Answer from the drawing. Dimensions are ordinates in mm from the lowest x, y and z of the part. A direction names the side the tool comes from. Coordinates: 2 decimals unless noted, no trailing zeros. Write each loop counter-clockwise with the first axis right and the second up, starting at its lowest first coordinate (ties: lowest second). Pieces come first, ordered by that corner, then holes. Notation, with made-up numbers: (36.5, 45.25) - (42.5, 45.25) arc R21 cw to (42.5, 56.25) - close; hole circle Ø6 at (-16, 29.5). An arc over 180 degrees is marked (long way). Use one line per item in the form item = value. Start each with the question number.
Item 1: A cutting plane is placed at D-D (z = 4). Write down the section's boundary in (x, y), then the cut area to 3 significant figures.
Item 2: Given pin 1 (4.5 mm diameter, centred on x = 6.5, y = 21.5, fed in from -Z); pin 2 (3.5 mm diameter, centred on x = 30.13, z = 32, fed in from -Y); pin 3 (5 mm diameter, centred on x = 28.5, z = 15.5, fed in from +Y); pin 4 (5 mm diameter, centred on y = 24, z = 29, fed in from +X), each flat-ended and moving along its own axis, determine where each tip first touches the part or whether it passes through.
Item 3: For the marked faces 4, 5 and 6, determine the directions among +Z, -Z, +X, -X, +Y, -Y from which every point of the face is accessible in a straight line to the end or side of a thin tool.
Item 4: A cutting plane is placed at B-B (x = 14). Write down the section's boundary in (y, z), then the cut area to 3 significant figures.
Item 5: A cutting plane is placed at C-C (y = 17). Write down the section's boundary in (x, z).
Item 6: Consider probe 1 along Y at (x, z) = (5, 27); probe 2 along X at (y, z) = (7, 32); probe 3 along X at (y, z) = (17, 14.5). Determine where each line is inside the solid, lowest interval first.
Item 7: A cutting plane is placed at A-A (z = 8). Write down the section's boundary in (x, y), then the cut area to 3 significant figures.
Item 8: Determine the mould class of the marked faces 1, 2 and 3 for opening direction Y: released by +Y, released by -Y, zero draft, split by the parting line, or undercut.
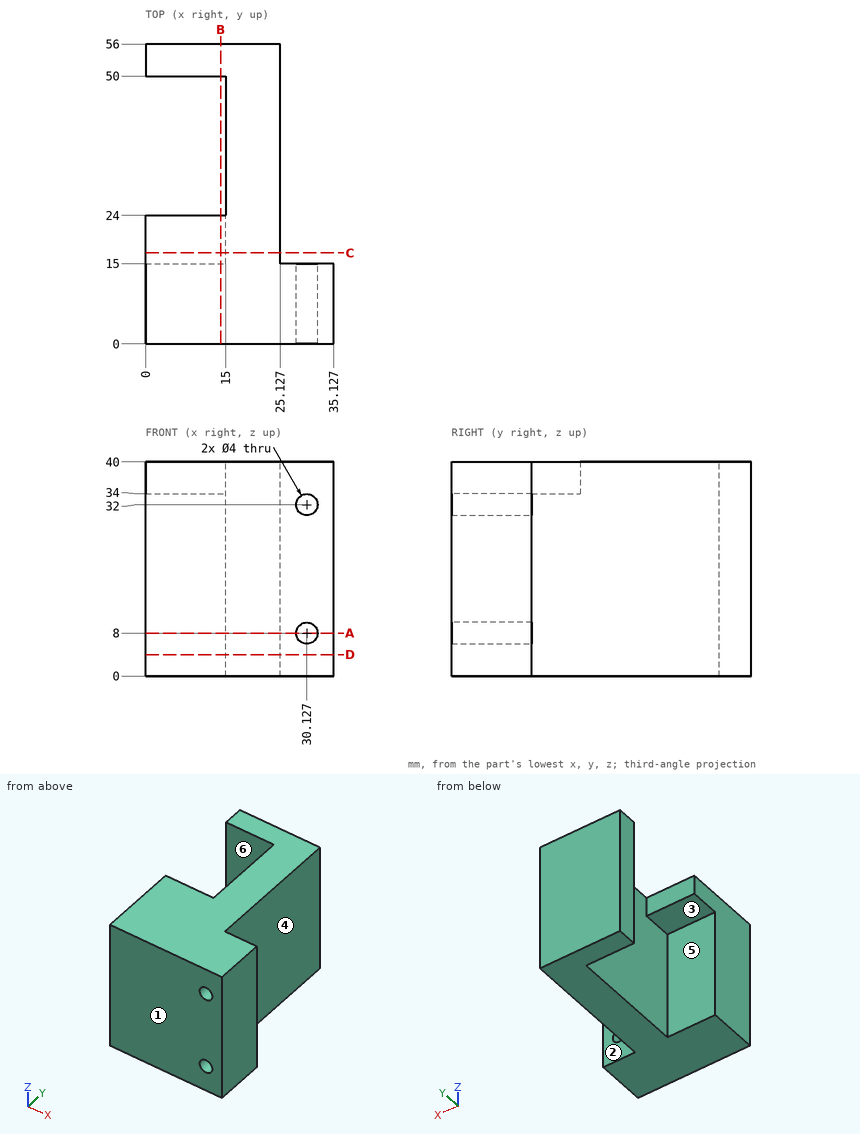
Answer:
q1.outline = (0, 0) - (35.13, 0) - (35.13, 15) - (25.13, 15) - (25.13, 56) - (0, 56) - (0, 50) - (15, 50) - (15, 15) - (0, 15) - close
q1.area = 1,030 mm²
q2.pin_1 = 34
q2.pin_2 = through
q2.pin_3 = 15
q2.pin_4 = 25.13
q3.face_4 = +Z, -Z, +X, +Y
q3.face_5 = -Z, -X
q3.face_6 = +Z, -Z, -X
q4.outline = (0, 0) - (15, 0) - (15, 34) - (24, 34) - (24, 40) - (0, 40) - close; (50, 0) - (56, 0) - (56, 40) - (50, 40) - close
q4.area = 894 mm²
q5.outline = (0, 34) - (15, 34) - (15, 0) - (25.13, 0) - (25.13, 40) - (0, 40) - close
q6.probe_1 = 0 to 15, 50 to 56
q6.probe_2 = 0 to 28.13, 32.13 to 35.13
q6.probe_3 = 15 to 25.13
q7.outline = (0, 0) - (28.13, 0) - (28.13, 15) - (25.13, 15) - (25.13, 56) - (0, 56) - (0, 50) - (15, 50) - (15, 15) - (0, 15) - close; (32.13, 0) - (35.13, 0) - (35.13, 15) - (32.13, 15) - close
q7.area = 972 mm²
q8.face_1 = released by -Y
q8.face_2 = released by +Y
q8.face_3 = undercut
